Model file for the job. Use its own axes, mm. Face numbers are marked on the shaded views. A direction names the side the tool comes from. Coordinates: 2 decimals unless noted, no trailing zeros. Write each loop counter-clockwise with the first axis right and the second up, starting at its lowest first coordinate (ties: lowest second). Pieces come first, ordered by that corner, then holes. Notation, with made-up numbers: M 69,-21.75 L 74,-21.75 A16 cw 74,-12.75 Z; hole C -35.75,-11 d11. An arc over 180 degrees is marked long. Answer in a Markdown table with one row per item. Add a question column.
```python
from build123d import *

# Parameters (mm, degrees)
SKETCH1_R           = 8
BOSS_EXTRUDE1_DEPTH = 50
SKETCH2_R           = 10
BOSS_EXTRUDE2_DEPTH = 35
SKETCH5_W           = 48
SKETCH5_H           = 42.813252044
CUT_EXTRUDE1_DEPTH  = 35


with BuildPart() as part:
    # Sketch1 → Boss-Extrude1 (new body, symmetric)
    with BuildSketch(Plane(origin=(0, 0, 0), x_dir=(0, 0, -1), z_dir=(1, 0, 0))):
        Circle(SKETCH1_R)
    extrude(amount=BOSS_EXTRUDE1_DEPTH, both=True)

    # Sketch2 → Boss-Extrude2 (add, symmetric)
    with BuildSketch(Plane(origin=(0, 0, 0), x_dir=(0, 0, -1), z_dir=(1, 0, 0))):
        with BuildLine():
            Line((-11, -15), (11, -15))
            ThreePointArc((11, -15), (15.242640687, -13.242640687), (17, -9))
            Line((17, -9), (17, 25))
            ThreePointArc((17, 25), (0, 42), (-17, 25))
            Line((-17, 25), (-17, -9))
            ThreePointArc((-17, -9), (-15.242640687, -13.242640687), (-11, -15))
        make_face()
        with Locations((0, 25)):
            Circle(SKETCH2_R, mode=Mode.SUBTRACT)
    extrude(amount=BOSS_EXTRUDE2_DEPTH, both=True)

    # Sketch5 → Cut-Extrude1 (cut, through all)
    with BuildSketch(Plane.XY.offset(17)):
        with Locations((0, 20.593373978)):
            Rectangle(SKETCH5_W, SKETCH5_H)
    extrude(amount=-CUT_EXTRUDE1_DEPTH, mode=Mode.SUBTRACT)


solid = part.part
```
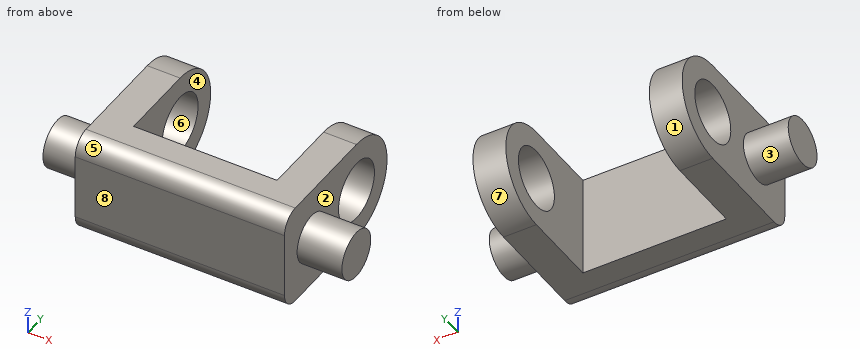
1) Drill centre lines: probe 1 along X at (y, z) = (17, -8); probe 2 along Z at (x, y) = (-28.5, 25); probe 3 along Y at (x, z) = (29, 0). Where is each one in solid material? Low to high.
2) Slice it at D-D (x = 8.5). Give the cut face in (y, z), then the cut area to 3 significant figures.
3) Flat gauge pins, fed straight in: pin 1 Ø1.5 at (y, z) = (-8, 5.5) entering from -X; pin 2 Ø4 at (x, z) = (38.5, 3.5) entering from +Y; pin 3 Ø10 at (x, z) = (-7, -2.5) entering from +Y. Where does each tip first touch, or does it go through?
4) Slice it at C-C (y = 34). Give the cut face in (x, z).
5) Which spindle directions (+Z, -Z, +X, -X, +Y, -Y) get a long thin tool onto all of the face, cutting with end or side? Do the marked faces 1, 2, 3, 4 and 5. Say none if no direction does.
6) Slice it at A-A (z = 0). Give the cut face in (x, y), then the cut area to 3 significant figures.
7) Two-plate mould, pull along Z, no slides. Class the marked faces 6, 7 and 8: released by +Z, released by -Z, zero draft, split by the parting line, or undercut.
8) Slice it at B-B (y = 7). Give the cut face in (x, z), then the cut area to 3 significant figures.
Ans:
| question | item | result |
|---|---|---|
| 1 | probe 1 | x = -35 to -24, 24 to 35 |
| 1 | probe 2 | z = -17 to -10, 10 to 17 |
| 1 | probe 3 | y = -15 to 15, 35 to 42 |
| 2 | outline | M -15,-11 A6 ccw -9,-17 L -0.81,-17 L -0.81,17 L -9,17 A6 ccw -15,11 Z |
| 2 | area | 467 mm2 |
| 3 | pin 1 | stops at x = -35 |
| 3 | pin 2 | stops at y = 7.86 |
| 3 | pin 3 | stops at y = -0.81 |
| 4 | outline | M -35,-14.42 L -24,-14.42 L -24,-4.36 L -35,-4.36 Z; M -35,4.36 L -24,4.36 L -24,14.42 L -35,14.42 Z; M 24,-14.42 L 35,-14.42 L 35,-4.36 L 24,-4.36 Z; M 24,4.36 L 35,4.36 L 35,14.42 L 24,14.42 Z |
| 5 | face 1 | +X, -X, +Y |
| 5 | face 2 | +X |
| 5 | face 3 | -X |
| 5 | face 4 | +Z, -Z, +Y |
| 5 | face 5 | +Z, +X, -X, -Y |
| 6 | outline | M -50,-8 L -35,-8 L -35,-15 L 35,-15 L 35,-8 L 50,-8 L 50,8 L 35,8 L 35,15 L 24,15 L 24,-0.81 L -24,-0.81 L -24,15 L -35,15 L -35,8 L -50,8 Z; M -35,35 L -24,35 L -24,42 L -35,42 Z; M 24,35 L 35,35 L 35,42 L 24,42 Z |
| 6 | area | 1,970 mm2 |
| 7 | face 6 | undercut |
| 7 | face 7 | split by the parting line |
| 7 | face 8 | zero draft |
| 8 | outline | M -50,-3.87 L -35,-3.87 L -35,-17 L -24,-17 L -24,17 L -35,17 L -35,3.87 L -50,3.87 Z; M 24,-17 L 35,-17 L 35,-3.87 L 50,-3.87 L 50,3.87 L 35,3.87 L 35,17 L 24,17 Z |
| 8 | area | 980 mm2 |
